Design review of the part built by this model. Coordinates are the model's own, in mm. A direction names the side the tool comes from. Give positions to 0.01 mm unless a question says otherwise; leave off trailing zeros. Write each loop counter-clockwise with the first axis right and the second up, starting at its lowest first coordinate (ties: lowest second). Pieces come first, ordered by that corner, then holes. Notation, with made-up numbers: M 35.5,15 L 91.5,15 A17 ccw 91.5,25 Z; hole C -17.5,87.25 d5. An arc over 180 degrees is marked long. Use a Markdown table: item, result. Add a question column.
```python
from build123d import *

# Parameters (mm, degrees)
SKETCH_1_R      = 1.7
SKETCH_1_R_2    = 3
SKETCH_1_R_3    = 4.1
EXTRUDE_1_DEPTH = 4


with BuildPart() as part:
    # 草图1 → 凸台-拉伸1 (new body)
    with BuildSketch(Plane.XY.offset(4)):
        with BuildLine():
            Line((40, -6), (70, -6))
            ThreePointArc((70, -6), (76.000000116, 1.16e-07), (70, 6.000000233))
            Line((70, 6.000000233), (39.999998847, 6.000000233))
            ThreePointArc((39.999998847, 6.000000233), (19.900249653, 7.002487606), (2.882e-06, 9.999999418))
            ThreePointArc((2.882e-06, 9.999999418), (-9.999999709, 1.15e-06), (0, -10))
            ThreePointArc((0, -10), (19.900248758, -7.002487578), (40, -6))
        make_face()
        with Locations(Location((0, 7, 0), (0, 0, 180))):
            Circle(SKETCH_1_R, mode=Mode.SUBTRACT)
        with Locations(Location((0, -2.91e-07, 0), (0, 0, 180))):
            Circle(SKETCH_1_R_2, mode=Mode.SUBTRACT)
        with Locations(Location((-7, 0, 0), (0, 0, 180))):
            Circle(SKETCH_1_R, mode=Mode.SUBTRACT)
        with Locations(Location((0, -7, 0), (0, 0, 180))):
            Circle(SKETCH_1_R, mode=Mode.SUBTRACT)
        with Locations(Location((7, 0, 0), (0, 0, 180))):
            Circle(SKETCH_1_R, mode=Mode.SUBTRACT)
        with Locations(Location((70, 1.16e-07, 0), (0, 0, 180))):
            Circle(SKETCH_1_R_3, mode=Mode.SUBTRACT)
    extrude(amount=-EXTRUDE_1_DEPTH)


solid = part.part
```
(1) The part is to be moulded in two halves that separate along X. For faces 3 (the cylindrical face through (20.181, 6.975, 2.028)), 4 (the flat face through (55, -6, 2)), 5 (the cylindrical face through (0.37, 8.66, 2.03)), say which applies: released by +X, released by -X, zero draft, split by the parting line, or undercut.
(2) Wall thickness on L1, parallel to X at y = -1.75, z = 1.6; L2, parallel to X at y = 2, z = 2.05; L3, parallel to X at y = 0.5, z = 1.65: over which ranges is each line inside the solid? List them lowest first.
(3) For pin 1 (1.5 mm diameter, centred on x = 31.5, y = -4, fed in from -Z); pin 2 (3.5 mm diameter, centred on x = 0, y = 0, fed in from +Z); pin 3 (1.2 mm diameter, centred on x = 52, z = 1, fed in from +Y), all flat-tipped, find the tip position at first contact; note any pin that passes through.
(4) Machinability: for faces 1 (the cylindrical face through (-2.86, -0.9, 2.03)), 2 (the flat face through (55, 6, 2)), which of the approach directions +Z, -Z, +X, -X, +Y, -Y give a long, thin tool a straight path to every point of the face, cutting with its end or side? Answer none if there is none.
(5) Add section A-A on y = 0. Give the boundary of the cut face in (x, z).
(6) Add section D-D on y = -7. Give the boundary of the cut face in (x, z), then the cut area to 3 significant figures.
(7) Add section B-B on x = -7. Give the boundary of the cut face in (y, z), then the cut area to 3 significant figures.
(8) Add section C-C on z = 1.6. Give the boundary of the cut face in (x, y).
From the geometry:
| question | item | result |
|---|---|---|
| 1 | face 3 | released by +X |
| 1 | face 4 | zero draft |
| 1 | face 5 | undercut |
| 2 | L1 | x = -9.85 to -2.44, 2.44 to 66.29, 73.71 to 75.74 |
| 2 | L2 | x = -9.8 to -2.24, 2.24 to 66.42, 73.58 to 75.66 |
| 2 | L3 | x = -9.99 to -8.62, -5.38 to -2.96, 2.96 to 5.38, 8.62 to 65.93, 74.07 to 75.98 |
| 3 | pin 1 | stops at z = 0 |
| 3 | pin 2 | passes through |
| 3 | pin 3 | stops at y = 6 |
| 4 | face 1 | +Z, -Z |
| 4 | face 2 | +Z, -Z, +X, +Y |
| 5 | outline | M -10,0 L -8.7,0 L -8.7,4 L -10,4 Z; M -5.3,0 L -3,0 L -3,4 L -5.3,4 Z; M 3,0 L 5.3,0 L 5.3,4 L 3,4 Z; M 8.7,0 L 65.9,0 L 65.9,4 L 8.7,4 Z; M 74.1,0 L 76,0 L 76,4 L 74.1,4 Z |
| 6 | outline | M -7.14,0 L -1.7,0 L -1.7,4 L -7.14,4 Z; M 1.7,0 L 19.93,0 L 19.93,4 L 1.7,4 Z |
| 6 | area | 94.7 mm^2 |
| 7 | outline | M -7.14,0 L -1.7,0 L -1.7,4 L -7.14,4 Z; M 1.7,0 L 7.14,0 L 7.14,4 L 1.7,4 Z |
| 7 | area | 43.5 mm^2 |
| 8 | outline | M 0,-10 A202 cw 40,-6 L 70,-6 A6 ccw 70,6 L 40,6 A202 cw 0,10 A10 ccw Z; hole C -7,0 d3.4; hole C 0,0 d6; hole C 0,-7 d3.4; hole C 0,7 d3.4; hole C 7,0 d3.4; hole C 70,0 d8.2 |
